from build123d import *

# Parameters (mm, degrees)
F0_R          = 101.6
F0_R_2        = 97.536
F1_DEPTH      = 762
F2_W          = 254
F2_H          = 254
F3_DEPTH      = 4.7625
F5_DEPTH      = 127.001
F5_DEPTH_BACK = 127.001
F6_DEPTH      = 127.001
F6_DEPTH_BACK = 127.001


with BuildPart() as f1:
    # F0 (on Top) → F1 (new body)
    with BuildSketch(Plane.XY):
        Circle(F0_R)
        Circle(F0_R_2, mode=Mode.SUBTRACT)
    extrude(amount=F1_DEPTH)

    # F2 (on Top) → F3 (join)
    with BuildSketch(Plane.XY):
        Rectangle(F2_W, F2_H)
    extrude(amount=-F3_DEPTH)

    # F4 (on Right) → F5 (cut, two sides)
    with BuildSketch(Plane.YZ) as f5_sk:
        Polygon((-101.6, 688.041248), (101.6, 762), (-101.6, 762), align=None)
    extrude(amount=-F5_DEPTH, mode=Mode.SUBTRACT)
    extrude(f5_sk.sketch, amount=-F5_DEPTH_BACK, mode=Mode.SUBTRACT)

    # F4 (on Right) → F6 (cut, two sides)
    with BuildSketch(Plane.YZ) as f6_sk:
        Polygon((-101.6, 688.041248), (101.6, 762), (-101.6, 762), align=None)
    extrude(amount=F6_DEPTH, mode=Mode.SUBTRACT)
    extrude(f6_sk.sketch, amount=-F6_DEPTH_BACK, mode=Mode.SUBTRACT)


solid = f1.part
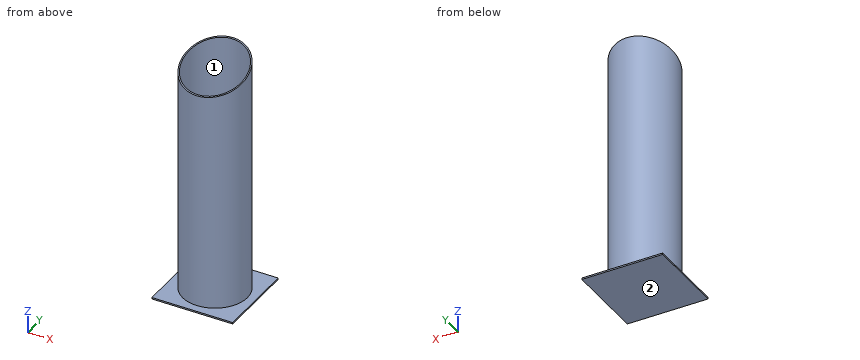
Geometry: final body of the model. Coordinates: model frame, mm. Face numbers are marked on the shaded views. A direction names the side the tool comes from. Coordinates: 2 decimals unless noted, no trailing zeros. Order: outer loops, then holes, each group sorted by start corner. A loop starts at its lowest first (then second) coordinate and runs counter-clockwise, first axis right, second up.
(1) Section query C-C (z = 441). Return the cut outline in (x, y).
(2) Access query for the marked faces 1 and 2. Directions: +Z, -Z, +X, -X, +Y, -Y. A direction counts if a zero-diameter tool reaches every point of the face in a straight line with its end or side. Return the directions, or none.
(3) Material intervals for probe 1 along Y at (x, z) = (0, 260); probe 2 along Z at (x, y) = (98.5, -77.5), sorted ascending.
(4) Section query B-B (y = 37.5). Return the cut outline in (x, z), plus the area to 3 significant figures.
(5) Section query A-A (x = 0). Return the cut outline in (y, z), plus the area to 3 significant figures.
(6) First-contact query: pin 1 (6 mm diameter, centred on x = 54, z = 459.5, fed in from -Y); pin 2 (1 mm diameter, centred on x = 88.5, y = 75, fed in from +Z); pin 3 (1 mm diameter, centred on x = 94.5, z = 155, fed in from -Y). Flat tips, straight axial feed; report the tip coordinate or a pass-through.
Solution:
1. outline: circle Ø203.2 at (0, 0); hole circle Ø195.07 at (0, 0)
2. face 1: +Z
2. face 2: -Z, +X, -X, +Y, -Y
3. probe 1: y = -101.6 to -97.54, 97.54 to 101.6
3. probe 2: z = -4.76 to 0
4. outline: (-127, -4.76) - (127, -4.76) - (127, 0) - (94.43, 0) - (94.43, 738.67) - (90.04, 738.67) - (90.04, 0) - (-90.04, 0) - (-90.04, 738.67) - (-94.43, 738.67) - (-94.43, 0) - (-127, 0) - close
4. area: 7,690 mm2
5. outline: (-127, -4.76) - (127, -4.76) - (127, 0) - (101.6, 0) - (101.6, 762) - (97.54, 760.52) - (97.54, 0) - (-97.54, 0) - (-97.54, 689.52) - (-101.6, 688.04) - (-101.6, 0) - (-127, 0) - close
5. area: 7,100 mm2
6. pin 1: stops at y = -87.87
6. pin 2: stops at z = 0
6. pin 3: stops at y = -38.56
